Autodesk Inventor part; units mm, degrees
ref_plane "YZ Plane" through (0, 0, 0) normal (1, 0, 0) x (0, 1, 0)
ref_plane "XZ Plane" through (0, 0, 0) normal (0, 1, 0) x (-1, 0, 0)
ref_plane "XY Plane" through (0, 0, 0) normal (0, 0, 1) x (1, 0, 0)
sketch "Szkic1" plane through (0, 0, 0) normal (0, 1, 0) x (-1, 0, 0)
  line L0 (0, 0) -> (42, 0)
  line L1 (42, 0) -> (42, -3)
  line L2 (42, -3) -> (0, -3)
  line L3 (0, -3) -> (0, 0)
  dimension "d0" = 42
  dimension "d1" = 3
extrude "Wyciągnięcie proste1" add sketch "Szkic1" along normal blind 8
sketch "Szkic2" plane through (0, 8, 0) normal (0, 1, 0) x (1, 0, 0)
  circle A0 centre (-39.3616, 1.5) radius 1
  point P0 (0, 0)
  dimension "d4" = 2
extrude "Wyciągnięcie proste2" cut sketch "Szkic2" against normal blind 0.2
sketch "Szkic3" plane through (0, 0, -3) normal (0, 0, -1) x (-1, 0, 0)
  line L0 (0, 0) -> (42, 0)
  line L1 (0, 8) -> (42, 8)
  line L2 (42, 0) -> (36, 0)
  line L3 (36, 0) -> (36, 8)
  line L4 (36, 8) -> (42, 8)
  line L5 (42, 8) -> (42, 0)
  line L6 (0, 8) -> (6, 8)
  line L7 (6, 8) -> (6, 0)
  line L8 (6, 0) -> (0, 0)
  line L9 (0, 0) -> (0, 8)
  circle A0 centre (9.5, 3) radius 0.85
  circle A1 centre (18.5, 3) radius 0.85
  circle A2 centre (23.5, 3) radius 0.85
  circle A3 centre (32.5, 3) radius 0.85
  circle A4 centre (14, 3) radius 1.95
  circle A5 centre (28, 3) radius 1.95
  dimension "d7" = 6
  dimension "d8" = 6
  dimension "d9" = 1.7
  dimension "d10" = 1.7
  dimension "d11" = 1.7
  dimension "d12" = 1.7
  dimension "d13" = 3.5
  dimension "d14" = 3.5
  dimension "d15" = 3
  dimension "d16" = 3
  dimension "d17" = 3
  dimension "d18" = 3
  dimension "d19" = 9
  dimension "d20" = 9
  dimension "d21" = 3.9
  dimension "d22" = 3
  dimension "d23" = 4.5
  dimension "d24" = 3.9
  dimension "d25" = 3
  dimension "d26" = 4.5
extrude "Wyciągnięcie proste3" cut sketch "Szkic3" against normal blind 3 contours A0 | A1 | A2 | A3 | A4 | A5
sketch "Szkic4" plane through (0, 8, 0) normal (0, 1, 0) x (1, 0, 0)
  line L0 (-42, 0) -> (0, 0)
  line L1 (-42, 0) -> (-36, 0)
  line L2 (-36, 0) -> (-36, 6)
  line L3 (-36, 6) -> (-42, 6)
  line L4 (-42, 6) -> (-42, 0)
  dimension "d29" = 6
  dimension "d30" = 6
extrude "Wyciągnięcie proste4" add sketch "Szkic4" against normal blind 8
sketch "Szkic5" plane through (0, 0, 0) normal (0, -1, 0) x (1, 0, 0)
  line L0 (-42, 0) -> (0, 0)
  line L1 (-36, -3) -> (-36, -6)
  line L2 (-42, 0) -> (-36, 0)
  line L3 (-36, 0) -> (-36, -6)
  line L4 (-36, -6) -> (-42, -6)
  line L5 (-42, -6) -> (-42, 0)
extrude "Wyciągnięcie proste5" cut sketch "Szkic5" against normal blind 3
sketch "Szkic20" plane through (0, 8, 0) normal (0, 1, 0) x (1, 0, 0)
  line L0 (0, 3) -> (-36, 3)
  line L1 (0, 0) -> (-6, 0)
  line L2 (-6, 0) -> (-6, 3)
  line L3 (-6, 3) -> (0, 3)
  line L4 (0, 3) -> (0, 0)
  line L5 (0, 0) -> (-6, 0)
  line L6 (-6, 0) -> (-6, 5.8)
  line L7 (-6, 5.8) -> (0, 5.8)
  line L8 (0, 5.8) -> (0, 0)
  line L9 (-6, 0) -> (2, 0)
  line L10 (2, 0) -> (2, -2.2)
  line L11 (2, -2.2) -> (-6, -2.2)
  line L12 (-6, -2.2) -> (-6, 0)
  line L13 (2, 0) -> (0, 0)
  line L14 (0, 0) -> (0, 5.8)
  line L15 (0, 5.8) -> (2, 5.8)
  line L16 (2, 5.8) -> (2, 0)
  dimension "d105" = 6
  dimension "d106" = 5.8
  dimension "d107" = 8
  dimension "d108" = 2.2
extrude "Wyciągnięcie proste23" add sketch "Szkic20" against normal blind 5
sketch "Szkic21" plane through (0, 0, 0) normal (0, -1, 0) x (1, 0, 0)
  line L0 (0, 0) -> (0, -3)
  line L1 (-6, 2.2) -> (-6, 0)
  line L2 (0, -3) -> (-6, -3)
  line L3 (-6, -3) -> (-6, 0)
  line L4 (-6, 0) -> (0, 0)
  line L5 (0, 0) -> (0, -3)
extrude "Wyciągnięcie proste24" cut sketch "Szkic21" against normal blind 3
sketch "Szkic22" plane through (0, 3, 0) normal (0, -1, 0) x (1, 0, 0)
  circle A0 centre (-2, -1.8) radius 2
  line L0 (-6, -5.8) -> (2, -5.8)
  line L1 (2, -5.8) -> (2, 2.2)
  line L2 (-6, -3) -> (-6, -5.8)
  line L3 (-6, -5.8) -> (2, -5.8)
  line L4 (2, -5.8) -> (2, -4.8)
  line L5 (2, -4.8) -> (-6, -4.8)
  line L6 (-6, -4.8) -> (-6, -5.8)
  line L7 (2, -4.8) -> (1, -4.8)
  line L8 (1, -4.8) -> (1, 2.2)
  line L9 (1, 2.2) -> (2, 2.2)
  line L10 (2, 2.2) -> (2, -4.8)
  line L11 (1, 2.2) -> (-6, 2.2)
  line L12 (-6, 2.2) -> (-6, 1.2)
  line L13 (-6, 1.2) -> (1, 1.2)
  line L14 (1, 1.2) -> (1, 2.2)
  point P0 (0, 0)
  point P1 (-2, -5.8)
  point P2 (2, -1.8)
  point P3 (2, 2.2)
  point P4 (1, 1.2)
  dimension "d113" = 4
  dimension "d114" = 4
  dimension "d115" = 4
  dimension "d116" = 8
  dimension "d117" = 1
  dimension "d118" = 1
  dimension "d119" = 1
extrude "Wyciągnięcie proste25" cut sketch "Szkic22" against normal blind 3.25 contours A0
extrude "Wyciągnięcie proste26" cut sketch "Szkic22" against normal blind 5 contours L2 L5 L1 L0 | L5 L8 L9 L1 | L13 L12 L11 L8
sketch "Szkic25" plane through (-42, 3, 0) normal (0, 0, 1) x (1, 0, 0)
  circle A0 centre (28, 0) radius 1.95
  circle A1 centre (28, 0) radius 2.2
  circle A2 centre (14, 0) radius 1.95
  circle A3 centre (14, 0) radius 2.2
  point P0 (42, -3)
  dimension "d132" = 4.4
  dimension "d133" = 4.4
extrude "Wyciągnięcie proste29" cut sketch "Szkic25" against normal blind 0.6 contours A0 | A1 | A2 | A3
sketch "Szkic26" plane through (0, 3, 0) normal (0, -1, 0) x (1, 0, 0)
  circle A0 centre (-39, -3) radius 2
  line L0 (-42, 0) -> (-36, 0)
  line L1 (-42, -6) -> (-42, 0)
  point P0 (0, 0)
  point P1 (-42, -3)
  dimension "d136" = 4
  dimension "d137" = 3
  dimension "d138" = 3
extrude "Wyciągnięcie proste30" cut sketch "Szkic26" against normal blind 4
fillet "Fillet1" radius 3 4 edges at (-42, 5.5, -6) (1, 5.5, -4.8) (-42, 5.5, 0) (1, 5.5, 1.2)
chamfer "Chamfer1" distance 0.4 angle 45 4 edges at (-31.65, 3, -3) (-22.65, 3, -3) (-17.65, 3, -3) (-8.65, 3, -3)
properties part number "rmwall" material "Tworzywo sztuczne PET"
Can you work these out from the model? Positions are in its coordinate system, mm. A direction names the side the tool comes from. Round coordinates to 2 decimals unless told otherwise and drop trailing zeros. Loops run counter-clockwise (first coordinate to the right, second up) from the corner with the lowest first, then second, coordinate; pieces in that order, holes last.
Item 1: Suppose I cut it at B-B, the plane x = -14. Write out the boundary of the cut face in (y, z), then the cut area to 3 significant figures.
Item 2: Which directions (+Z, -Z, +X, -X, +Y, -Y) give clear straight access to the entire face, cutting with the end or side of a thin tool? Please do faces 1 (the cylindrical face through (-2.434, 4.602, -3.752)), 2 (the flat face through (-21, 4, -3)), 3 (the flat face through (-22, 4, 0)), 4 (the flat face through (-4, 5, -4.8)).
Item 3: Suppose I cut it at A-A, the plane x = -23.5. Write out the boundary of the cut face in (y, z).
Item 4: Will these pins go through, and if not, where does the flat tip stop? pin 1 Ø2 at (x, y) = (-9.5, 3) entering from +Z; pin 2 Ø0.9 at (y, z) = (1, -2) entering from -X; pin 3 Ø1.5 at (y, z) = (1.5, -2) entering from +X; pin 4 Ø1.3 at (x, y) = (-27, 3.5) entering from +Z.
Item 5: Suppose I cut it at C-C, the plane z = -5.5. Write out the boundary of the cut face in (x, y), then the cut area to 3 significant figures.
Item 6: If we mould it in two halves opening along Y, with no side actions, what happens to faces 5 (the cylindrical face through (-29.86, 3.59, -1.82)), 6 (the cylindrical face through (-11.9, 3.66, -0.3)), 7 (the flat face through (-36, 1, -1)), 8 (the flat face through (-39, 7, -3))? For each: +Y half, -Y half, draft (parallel to the pull), parting line (faces both ways), or undercut.
Item 7: Suppose I cut it at D-D, the plane x = -7. Write out the boundary of the cut face in (y, z).
Item 8: Please list where these lines run through material, in increasing order: L1, parallel to Y at x = -14, z = -1.15; L2, parallel to X at y = 4, z = -4; L3, parallel to Z at x = -11.5, y = 0.5.
Reported:
1. outline: (0, -3) - (1.05, -3) - (1.05, -0.6) - (0.8, -0.6) - (0.8, 0) - (0, 0) - close; (4.95, -3) - (8, -3) - (8, 0) - (5.2, 0) - (5.2, -0.6) - (4.95, -0.6) - close
1. area: 12.0 mm2
2. face 1: -Y
2. face 2: -Z, +Y, -Y
2. face 3: +Z, -X, +Y, -Y
2. face 4: -Z, +X, +Y, -Y
3. outline: (0, -3) - (1.75, -3) - (2.15, -2.6) - (2.15, 0) - (0, 0) - close; (3.85, -2.6) - (4.25, -3) - (8, -3) - (8, 0) - (3.85, 0) - close
4. pin 1: stops at z = 0
4. pin 2: stops at x = -36
4. pin 3: stops at x = -6
4. pin 4: passes through
5. outline: (-40.66, 3) - (-36, 3) - (-36, 8) - (-40.66, 8) - close
5. area: 23.3 mm2
6. face 5: undercut
6. face 6: undercut
6. face 7: draft
6. face 8: -Y half
7. outline: (0, -3) - (8, -3) - (8, 0) - (0, 0) - close
8. L1: y = 0 to 1.05, 4.95 to 8
8. L2: x = -41.83 to -40.73, -37.27 to -36, -6 to 0.04
8. L3: z = -3 to 0
